from build123d import *

# Parameters (mm, degrees)
F0_R     = 0.9
F1_DEPTH = 6
F2_R     = 20
F2_R_2   = 0.5
F3_DEPTH = 3


with BuildPart() as f1:
    # F0 (on Right) → F1 (new body)
    with BuildSketch(Plane.YZ):
        Polygon((17.5, -6.9), (17.5, 5.6), (17.5, 6.9), (17.5, 8.1), (-17.5, 8.1), (-17.5, 6.9), (-17.5, -6.9), align=None)
        with Locations((-13.8, 0)):
            Circle(F0_R, mode=Mode.SUBTRACT)
        Polygon((11.4, 6.4), (11.4, 5.9), (11.4, -5.9), (-11.4, -5.9), (-11.4, 5.9), (-11.4, 6.4), align=None, mode=Mode.SUBTRACT)
        with Locations((13.8, 0)):
            Circle(F0_R, mode=Mode.SUBTRACT)
    extrude(amount=F1_DEPTH)

    # F2 (on face) → F3 (join)
    with BuildSketch(Plane(origin=(0, 0, -6.9), x_dir=(1, 0, 0), z_dir=(0, 0, -1))):
        Circle(F2_R)
        Circle(F2_R_2, mode=Mode.SUBTRACT)
    extrude(amount=F3_DEPTH)


solid = f1.part
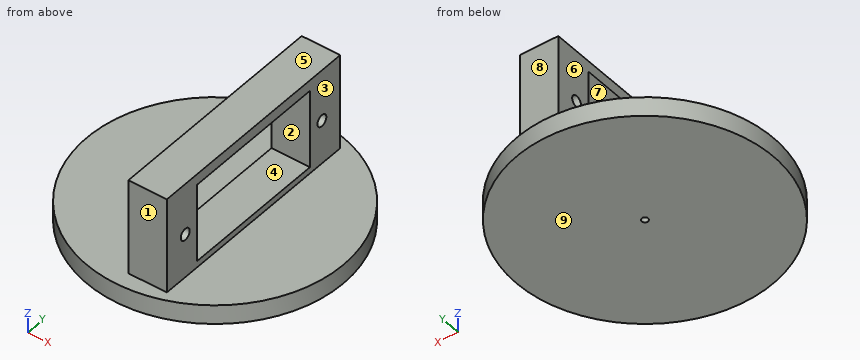
For this review, take the finished solid that the model builds, in its own axes (mm). Face numbers are marked on the shaded views. A direction names the side the tool comes from. Give positions to 0.01 mm unless a question says otherwise; leave off trailing zeros. Loops run counter-clockwise (first coordinate to the right, second up) from the corner with the lowest first, then second, coordinate; pieces in that order, holes last. Notation, with made-up numbers: M -1,34.5 L 30,34.5 A36 cw 30,73.5 Z; hole C 23,59.25 d2. An arc over 180 degrees is marked long. Answer as a JSON object with one key per item and string values. Group by question number.
Q1. For probe 1 along Y at (x, z) = (1, 3.75); probe 2 along Z at (x, y) = (2.7, -13.8); probe 3 along X at (y, z) = (0, -7.85), list the stretches that pass through material, from the lowest coordinate up. Write a range as [from, to].
Q2. Add section B-B on y = 0. Give the boundary of the cut face in (x, z).
Q3. Tool access review of the marked faces 5, 6, 7, 8 and 9: name each direction out of +Z, -Z, +X, -X, +Y, -Y from which nothing blocks a thin tool from reaching the whole face with its end or side.
Q4. Add section C-C on y = -13.5. Give the boundary of the cut face in (x, z), and give its area (3 significant figures).
Q5. Add section A-A on z = -4.5. Give the boundary of the cut face in (x, y).
Q6. Insertion check: P1, Ø10, axis at x = 1, z = -2.5, coming from the -Y side; P2, Ø1.5, axis at y = -7.5, z = 5, coming from the -X side; P3, Ø10, axis at x = -7.5, y = -8, coming from the +Z side; P4, Ø2.5, axis at y = -13.8, z = 0, coming from the +X side. Each pin has a flat end and moves straight along its axis. Give the tip position at first contact, or say it passes through.
Q7. Mouldability with a two-part tool opening along Y and no side actions: class the marked faces 1, 2, 3 and 4 as +Y half, -Y half, draft (parallel to the pull), parting line (faces both ways), or undercut.
Q8. Add section D-D on z = 0. Give the boundary of the cut face in (x, y), and give its area (3 significant figures).
Checked values:
{
 "1": {"probe 1": "[-17.5, -11.4], [11.4, 17.5]", "probe 2": "[-9.9, -0.9], [0.9, 8.1]", "probe 3": "[-20, -0.5], [0.5, 20]"},
 "2": {"outline": "M -20,-9.9 L -0.5,-9.9 L -0.5,-6.9 L -20,-6.9 Z; M 0,-6.9 L 0.5,-6.9 L 0.5,-9.9 L 20,-9.9 L 20,-6.9 L 6,-6.9 L 6,-5.9 L 0,-5.9 Z; M 0,6.4 L 6,6.4 L 6,8.1 L 0,8.1 Z"},
 "3": {"face 5": "+Z, +X, -X, +Y, -Y", "face 6": "+Z, -X, +Y, -Y", "face 7": "+X, -X", "face 8": "+Z, +X, -X, +Y", "face 9": "-Z, +X, -X, +Y, -Y"},
 "4": {"outline": "M -14.76,-9.9 L 14.76,-9.9 L 14.76,-6.9 L 6,-6.9 L 6,-0.85 L 0,-0.85 L 0,-6.9 L -14.76,-6.9 Z; M 0,0.85 L 6,0.85 L 6,8.1 L 0,8.1 Z", "area": "168 mm²"},
 "5": {"outline": "M 0,-17.5 L 6,-17.5 L 6,-11.4 L 0,-11.4 Z; M 0,11.4 L 6,11.4 L 6,17.5 L 0,17.5 Z"},
 "6": {"P1": "y = -20", "P2": "through", "P3": "z = -6.9", "P4": "x = 6"},
 "7": {"face 1": "-Y half", "face 2": "undercut", "face 3": "draft", "face 4": "undercut"},
 "8": {"outline": "M 0,-17.5 L 6,-17.5 L 6,-14.7 L 0,-14.7 Z; M 0,-12.9 L 6,-12.9 L 6,-11.4 L 0,-11.4 Z; M 0,11.4 L 6,11.4 L 6,12.9 L 0,12.9 Z; M 0,14.7 L 6,14.7 L 6,17.5 L 0,17.5 Z", "area": "51.6 mm²"}
}
